Here's the drawing with two shaded views (mm, measured from the low corner). I have some questions. A direction names the side the tool comes from. Round coordinates to 2 decimals unless told otherwise and drop trailing zeros. Loops run counter-clockwise (first coordinate to the right, second up) from the corner with the lowest first, then second, coordinate; pieces in that order, holes last. Notation, with made-up numbers: (88, -9) -> (132, -9) arc R34 ccw to (132, 21) -> close; hole circle Ø1 at (25.5, 81.5). An arc over 180 degrees is marked (long way). Write item = value, one per line.
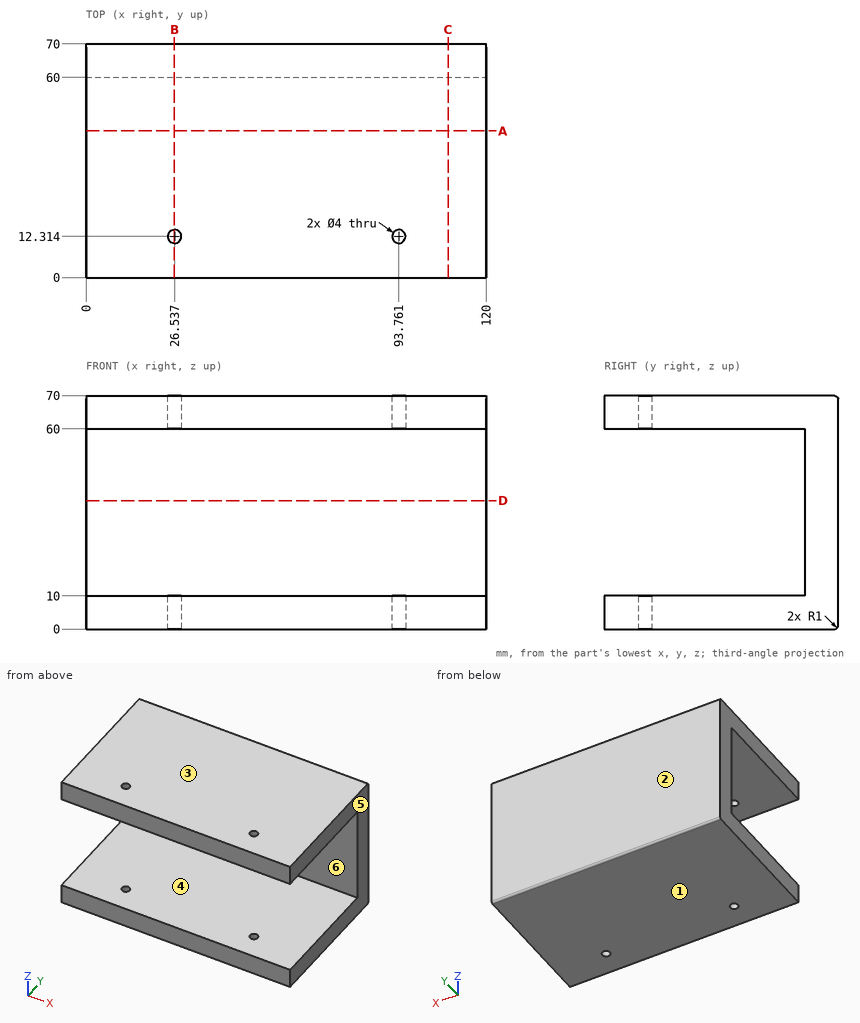
1. Suppose I cut it at A-A, the plane y = 44. List the corners of the cut face in (x, z) for me.
Entries:
outline = (0, 0) -> (120, 0) -> (120, 10) -> (0, 10) -> close; (0, 60) -> (120, 60) -> (120, 70) -> (0, 70) -> close
2. I need wall thicknesses on line 1 (Z direction, x = 83.5, y = 36.5); line 2 (Y direction, x = 75.5, z = 58.5). Which ranges of each line are inside material? Lowest first, please. Write a range as [from, to].
Entries:
line_1 = [0, 10], [60, 70]
line_2 = [60, 70]
3. I'm going to push flat-ended pins straight in: pin 1 (8 mm diameter, centred on x = 48.5, z = 55.5, fed in from -Y); pin 2 (1 mm diameter, centred on y = 58, z = 36, fed in from +X). Where does each tip first touch, or does it pass through?
Entries:
pin_1 = 60
pin_2 = through
4. Suppose I cut it at C-C, the plane x = 108.5. List the corners of the cut face in (y, z) for me, and give its area (3 significant figures).
Entries:
outline = (0, 0) -> (69, 0) arc R1 ccw to (70, 1) -> (70, 69) arc R1 ccw to (69, 70) -> (0, 70) -> (0, 60) -> (60, 60) -> (60, 10) -> (0, 10) -> close
area = 1,900 mm²
5. Suppose I cut it at B-B, the plane x = 26.5. List the corners of the cut face in (y, z) for me, and give its area (3 significant figures).
Entries:
outline = (0, 0) -> (10.31, 0) -> (10.31, 10) -> (0, 10) -> close; (0, 60) -> (10.31, 60) -> (10.31, 70) -> (0, 70) -> close; (14.31, 0) -> (69, 0) arc R1 ccw to (70, 1) -> (70, 69) arc R1 ccw to (69, 70) -> (14.31, 70) -> (14.31, 60) -> (60, 60) -> (60, 10) -> (14.31, 10) -> close
area = 1,820 mm²
6. Suppose I cut it at D-D, the plane z = 38.5. List the corners of the cut face in (x, y) for me, and give its area (3 significant figures).
Entries:
outline = (0, 60) -> (120, 60) -> (120, 70) -> (0, 70) -> close
area = 1,200 mm²
7. We'd pull the mould along Z, two halves only. Please class the marked faces 1, 2, 3 and 4: released by +Z, released by -Z, zero draft, split by the parting line, or undercut.
Entries:
face_1 = released by -Z
face_2 = zero draft
face_3 = released by +Z
face_4 = undercut
8. For the marked faces 5 and 6, which set-ups out of +Z, -Z, +X, -X, +Y, -Y let a thin tool reach every point of the face, with its end or its side?
Entries:
face_5 = +Z, -Z, +X, +Y, -Y
face_6 = +X, -X, -Y
